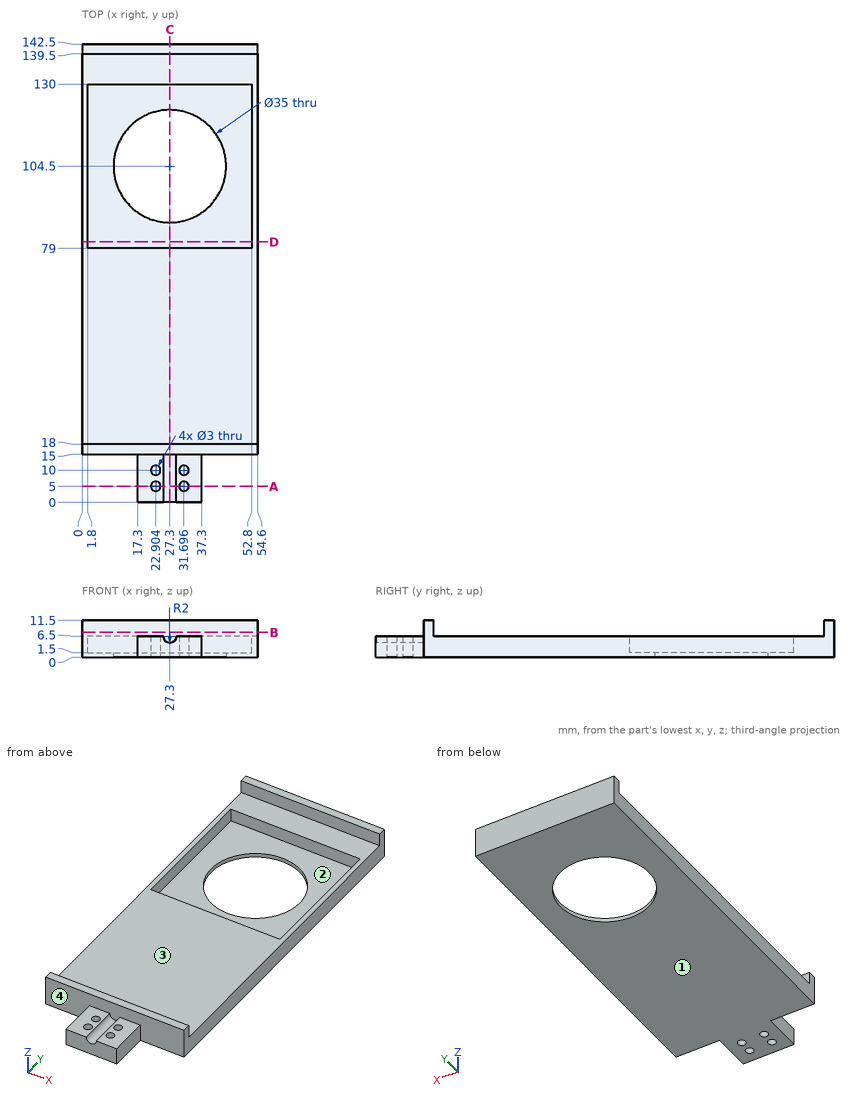
Drawing for the job (mm, zero at the part's lowest x, y, z). Give positions to 0.01 mm unless a question says otherwise; leave off trailing zeros. Loops run counter-clockwise (first coordinate to the right, second up) from the corner with the lowest first, then second, coordinate; pieces in that order, holes last.
(1) Pull direction Y, two halves, no side cores. Call the marked faces 1, 2, 3 and 4: pulls with the +Y half, pulls with the -Y half, needs draft (parallel to the pull), parting line crosses it, or undercut.
Return value:
face 1: needs draft
face 2: undercut
face 3: undercut
face 4: pulls with the -Y half
(2) Band-saw the part on A-A (y = 5). Write the cut outline in (x, z).
Return value:
outline: (17.3, 0) - (21.4, 0) - (21.4, 6.5) - (17.3, 6.5) - close; (24.4, 0) - (30.2, 0) - (30.2, 6.5) - (29.3, 6.5) arc R2 cw to (25.3, 6.5) - (24.4, 6.5) - close; (33.2, 0) - (37.3, 0) - (37.3, 6.5) - (33.2, 6.5) - close
(3) Band-saw the part on C-C (x = 27.3). Write the cut outline in (y, z), and give its area (3 significant figures).
Return value:
outline: (0, 0) - (87, 0) - (87, 1.5) - (79, 1.5) - (79, 6.5) - (18, 6.5) - (18, 11.5) - (15, 11.5) - (15, 4.5) - (0, 4.5) - close; (122, 0) - (142.5, 0) - (142.5, 11.5) - (139.5, 11.5) - (139.5, 6.5) - (130, 6.5) - (130, 1.5) - (122, 1.5) - close
area: 619 mm2
(4) Pin check, flat tips, straight feed: pin 1 (9 mm diameter, centred on x = 23, y = 8.5, fed in from +Z); pin 2 (5 mm diameter, centred on x = 43, z = 2.5, fed in from -Y); pin 3 (5 mm diameter, centred on y = 36, z = 6, fed in from -X); pin 4 (16.5 mm diameter, centred on x = 19, y = 88, fed in from +Z). Stop position of each tip, or through.
Return value:
pin 1: stops at z = 6.5
pin 2: stops at y = 15
pin 3: stops at x = 0
pin 4: stops at z = 1.5
(5) Drill centre lines: line 1 along X through (y, z) = (86, 3); line 2 along Y through (x, z) = (25, 4.5); line 3 along Y through (x, z) = (51, 3.5). Where is each one in solid material? Low to high.
Return value:
line 1: x = 0 to 1.8, 52.8 to 54.6
line 2: y = 0 to 79, 130 to 142.5
line 3: y = 15 to 79, 130 to 142.5
(6) Band-saw the part on D-D (y = 81). Write the cut outline in (x, z).
Return value:
outline: (0, 0) - (54.6, 0) - (54.6, 6.5) - (52.8, 6.5) - (52.8, 1.5) - (1.8, 1.5) - (1.8, 6.5) - (0, 6.5) - close
(7) Band-saw the part on B-B (z = 7.75). Write the cut outline in (x, y).
Return value:
outline: (0, 15) - (54.6, 15) - (54.6, 18) - (0, 18) - close; (0, 139.5) - (54.6, 139.5) - (54.6, 142.5) - (0, 142.5) - close
